Source: CAD feature listing. Evaluate the final solid. Frame: model axes, mm. Face numbers are marked on the shaded views. A direction names the side the tool comes from. Coordinates: 2 decimals unless noted, no trailing zeros. Write each loop counter-clockwise with the first axis right and the second up, starting at its lowest first coordinate (ties: lowest second). Pieces come first, ordered by that corner, then holes. Notation, with made-up numbers: (-21, 73) -> (-4, 73) arc R26 ccw to (-4, 109) -> close; hole circle Ø6 at (-33, -14.5). An arc over 180 degrees is marked (long way). Write item = value, one per line.
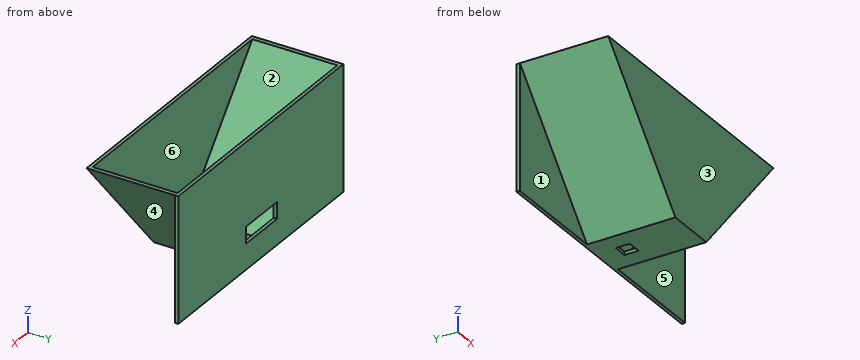
from build123d import *

# Parameters (mm, degrees)
BOSS_EXTRUDE1_DEPTH = 55
SHELL1_T            = -2
SKETCH6_W           = 30
SKETCH6_H           = 10.709947061
CUT_EXTRUDE3_DEPTH  = 4
SKETCH5_W           = 8.5
SKETCH5_H           = 8.497801987
CUT_EXTRUDE5_DEPTH  = 6
SKETCH10_W          = 160
SKETCH10_H          = 2
BOSS_EXTRUDE2_DEPTH = 75
SKETCH11_W          = 30
SKETCH11_H          = 10
CUT_EXTRUDE6_DEPTH  = 8


with BuildPart() as part:
    # Sketch1 → Boss-Extrude1 (new body)
    with BuildSketch(Plane(origin=(0, 0, 0), x_dir=(1, 0, 0), z_dir=(0, 1, 0))):
        Polygon((0, 0), (-160, 0), (-94.996692416, 75), (-64.996692416, 75), align=None)
    extrude(amount=-BOSS_EXTRUDE1_DEPTH)

    # Shell1
    shell1_openings = [part.faces().sort_by_distance(p)[0] for p in [
        (-80, -27.5, 0),
    ]]
    offset(amount=SHELL1_T, openings=shell1_openings, kind=Kind.INTERSECTION)

    # Sketch6 → Cut-Extrude3 (cut)
    with BuildSketch(Plane(origin=(0, 0, 0), x_dir=(1, 0, 0), z_dir=(0, 1, 0))):
        with Locations((-80.447039031, 51.579276021)):
            Rectangle(SKETCH6_W, SKETCH6_H)
    extrude(amount=-CUT_EXTRUDE3_DEPTH, mode=Mode.SUBTRACT)

    # Sketch5 → Cut-Extrude5 (cut)
    with BuildSketch(Plane.XY.offset(-73)):
        with Locations((-79.998465085, -16.748900994)):
            Rectangle(SKETCH5_W, SKETCH5_H)
    extrude(amount=-CUT_EXTRUDE5_DEPTH, mode=Mode.SUBTRACT)

    # Sketch10 → Boss-Extrude2 (add)
    with BuildSketch(Plane.XY):
        with Locations((-80, -1)):
            Rectangle(SKETCH10_W, SKETCH10_H)
    extrude(amount=-BOSS_EXTRUDE2_DEPTH)

    # Sketch11 → Cut-Extrude6 (cut)
    with BuildSketch(Plane(origin=(0, -2, 0), x_dir=(-1, 0, 0), z_dir=(0, -1, 0))):
        with Locations((80.729529252, 54.69995574)):
            Rectangle(SKETCH11_W, SKETCH11_H)
    extrude(amount=-CUT_EXTRUDE6_DEPTH, mode=Mode.SUBTRACT)


solid = part.part
1) Cut plane D-D, the plane x = -43.5. Output: boundary loops of the cut face in (y, z), and give its area (3 significant figures).
Answer block:
outline = (-55, -50.19) -> (-2, -50.19) -> (-2, -75) -> (0, -75) -> (0, 0) -> (-2, 0) -> (-2, -47.14) -> (-53, -47.14) -> (-53, 0) -> (-55, 0) -> close
area = 406 mm2
2) Pull-direction query (X, two-part tool) for the marked faces 4, 5 and 6; classes: +X half, -X half, draft (parallel to the pull), parting line (faces both ways), or undercut.
Answer block:
face_4 = +X half
face_5 = draft
face_6 = undercut
3) Cut plane C-C, the plane z = -13. Output: boundary loops of the cut face in (x, y), and give its area (3 significant figures).
Answer block:
outline = (-160, -2) -> (-148.73, -2) -> (-148.73, -55) -> (-11.27, -55) -> (-11.27, -2) -> (0, -2) -> (0, 0) -> (-160, 0) -> close; hole (-146.09, -53) -> (-13.91, -53) -> (-13.91, -2) -> (-146.09, -2) -> close
area = 865 mm2
4) First-contact query: pin 1 Ø6 at (x, y) = (-112.5, -31.5) entering from +Z; pin 2 Ø14 at (x, y) = (-83, -28) entering from +Z; pin 3 Ø1 at (y, z) = (-18, -74.5) entering from -X. Flat tips, straight axial feed; report the tip coordinate or a pass-through.
Answer block:
pin_1 = -48.29
pin_2 = -73
pin_3 = -95.86
5) Reachability of the marked faces 1, 2 and 3 from +Z, -Z, +X, -X, +Y, -Y: full face, straight path, thin tool, end or side. Return the list, or none.
Answer block:
face_1 = -Z, -X, -Y
face_2 = +Z
face_3 = +Z, -Z, +X, -X, -Y
6) Cut plane A-A, the plane x = -72. Output: boundary loops of the cut face in (y, z).
Answer block:
outline = (-55, -75) -> (0, -75) -> (0, -59.7) -> (-2, -59.7) -> (-2, -73) -> (-53, -73) -> (-53, 0) -> (-55, 0) -> close; (-2, -49.7) -> (0, -49.7) -> (0, 0) -> (-2, 0) -> close
7) Cut plane B-B, the plane y = -17.5. Output: boundary loops of the cut face in (x, z), and give its area (3 significant figures).
Answer block:
outline = (-160, 0) -> (-95, -75) -> (-84.25, -75) -> (-84.25, -73) -> (-94.08, -73) -> (-157.35, 0) -> close; (-75.75, -75) -> (-65, -75) -> (0, 0) -> (-2.65, 0) -> (-65.91, -73) -> (-75.75, -73) -> close
area = 433 mm2
8) Material intervals for probe 1 along Y at (x, z) = (-118, -43.5); probe 2 along Z at (x, y) = (-76, -3); probe 3 along X at (y, z) = (-18.5, -59), sorted ascending. Write a range as [from, to].
Answer block:
probe_1 = [-55, -53], [-2, 0]
probe_2 = [-75, -73]
probe_3 = [-108.86, -106.22], [-53.78, -51.13]
